For this review, take the finished solid that the model builds, in its own axes (mm). A direction names the side the tool comes from. Round coordinates to 2 decimals unless told otherwise and drop trailing zeros. Loops run counter-clockwise (first coordinate to the right, second up) from the corner with the lowest first, then second, coordinate; pieces in that order, holes last. Notation, with made-up numbers: (26, -26) -> (54, -26) arc R18 ccw to (54, -9) -> close; hole circle Ø3 at (58.5, -37). An arc over 180 degrees is marked (long way). One line per question, with ' | ' between items. Start each with the question number.
1. Consider section D-D (z = 1.5). Write out the cut boundary in (x, y), and give its area (3 significant figures).
2. Consider section C-C (y = 0). Write out the cut boundary in (x, z).
3. Consider section A-A (z = 5). Write out the cut boundary in (x, y).
4. Wall thickness on line 1 along Z through (x, y) = (6, -3); line 2 along Z through (x, y) = (13.5, -8); line 3 along Y through (x, z) = (0, 2.25): over which ranges is each line inside the solid? List them lowest first.
5. Draft analysis for pull direction X (two halves, no side actions). For faces 4 (the face through (14, -6, 2)), 5 (the face through (0, 0, 0)), state which applies: pulls with the +X half, pulls with the -X half, needs draft (parallel to the pull), parting line crosses it, or undercut.
6. For pin 1 Ø15 at (x, y) = (5.5, 4.5) entering from +Z; pin 2 Ø1.5 at (x, z) = (-9.5, 2) entering from -Y; pin 3 Ø2 at (x, z) = (9.5, 1.5) entering from +Y, all flat-tipped, find the tip position at first contact; note any pin that passes through.
7. For faces 1 (the face through (-12.1, -11.3, 4.5)), 2 (the face through (0, 0, 3)), 3 (the face through (12, -11.11, 7.51)), list the 3-axis set-ups (+Z, -Z, +X, -X, +Y, -Y) from which the entire face can be reached by the end or side of a thin tool; tool diameter is ignored.
8. Consider section B-B (x = 0). Write out the cut boundary in (y, z), and give its area (3 significant figures).
```python
from build123d import *

# Parameters (mm, degrees)
SKETCH1_R                                   = 17
SKETCH1_R_2                                 = 15
BOSS_EXTRUDE1_DEPTH                         = 2
SKETCH1_2_R                                 = 15
BOSS_EXTRUDE2_DEPTH                         = 3
BOSS_EXTRUDE3_DEPTH                         = 6
CUT_EXTRUDE1_START                          = -6
CUT_EXTRUDE1_DEPTH                          = 2.5
CHAMFER1_SIZE                               = 1
CHAMFER1_SIZE2                              = 0.2
CIRPATTERN1_COUNT                           = 2
CIRPATTERN1_ANGLE                           = 133
CHAMFER1_OF_CIRPATTERN1_SIZE2               = 0.2
CHAMFER1_OF_CIRPATTERN1_SIZE                = 1
CIRPATTERN1_THE_OTHER_WAY_COUNT             = 2
CIRPATTERN1_THE_OTHER_WAY_ANGLE             = 133
CHAMFER1_OF_CIRPATTERN1_THE_OTHER_WAY_SIZE2 = 0.2
CHAMFER1_OF_CIRPATTERN1_THE_OTHER_WAY_SIZE  = 1


with BuildPart() as part:
    # Sketch1 → Boss-Extrude1 (new body)
    with BuildSketch(Plane.XY):
        Circle(SKETCH1_R)
        Circle(SKETCH1_R_2, mode=Mode.SUBTRACT)
    extrude(amount=BOSS_EXTRUDE1_DEPTH)

    # Sketch1<2> → Boss-Extrude2 (add)
    with BuildSketch(Plane.XY):
        Circle(SKETCH1_2_R)
    extrude(amount=BOSS_EXTRUDE2_DEPTH)

    # Sketch2 → Boss-Extrude3 (add)
    with BuildSketch(Plane.XY.offset(2)):
        with BuildLine():
            ThreePointArc((4.184615385, 16.476923077), (0, 17), (-4.184615385, 16.476923077))
            Line((-4.184615385, 16.476923077), (-4, 15.75))
            ThreePointArc((-4, 15.75), (0, 16.25), (4, 15.75))
            Line((4, 15.75), (4.184615385, 16.476923077))
        make_face()
    boss_extrude3 = extrude(amount=BOSS_EXTRUDE3_DEPTH)

    # Sketch3 → Cut-Extrude1 (cut)
    with BuildSketch(Plane.XY.offset(8).offset(CUT_EXTRUDE1_START)):
        with BuildLine():
            ThreePointArc((1.25, 16.953981833), (0, 17), (-1.25, 16.953981833))
            Line((-1.25, 16.953981833), (-1.194852941, 16.206012046))
            ThreePointArc((-1.194852941, 16.206012046), (0, 16.25), (1.194852941, 16.206012046))
            Line((1.194852941, 16.206012046), (1.25, 16.953981833))
        make_face()
    cut_extrude1 = extrude(amount=CUT_EXTRUDE1_DEPTH, mode=Mode.SUBTRACT)

    # Chamfer1
    chamfer1_edges = [part.edges().sort_by_distance(p)[0] for p in [
        (0, 16.25, 8),
    ]]
    chamfer1_side = [part.faces().sort_by_distance(p)[0] for p in [
        (0, 16.25, 5),
    ]]
    chamfer(chamfer1_edges, length=CHAMFER1_SIZE, length2=CHAMFER1_SIZE2, reference=chamfer1_side[0])

    # CirPattern1: Boss-Extrude3, Cut-Extrude1 ×2 about axis
    cirpattern1_axis = Axis((0, 0, 0), (0, 0, -1))
    for i in range(1, CIRPATTERN1_COUNT):
        add(boss_extrude3.rotate(cirpattern1_axis, i * CIRPATTERN1_ANGLE / (CIRPATTERN1_COUNT - 1)))
        add(cut_extrude1.rotate(cirpattern1_axis, i * CIRPATTERN1_ANGLE / (CIRPATTERN1_COUNT - 1)), mode=Mode.SUBTRACT)

    # Chamfer1 of CirPattern1
    chamfer1_of_cirpattern1_edges = [part.edges().sort_by_distance(p)[0] for p in [
        (11.884497651, -11.082473351, 8),
    ]]
    chamfer(chamfer1_of_cirpattern1_edges, length=CHAMFER1_OF_CIRPATTERN1_SIZE, length2=CHAMFER1_OF_CIRPATTERN1_SIZE2)

    # CirPattern1 the other way: Boss-Extrude3, Cut-Extrude1 ×2 about axis
    cirpattern1_the_other_way_axis = Axis((0, 0, 0), (0, 0, 1))
    for i in range(1, CIRPATTERN1_THE_OTHER_WAY_COUNT):
        add(boss_extrude3.rotate(cirpattern1_the_other_way_axis, i * CIRPATTERN1_THE_OTHER_WAY_ANGLE / (CIRPATTERN1_THE_OTHER_WAY_COUNT - 1)))
        add(cut_extrude1.rotate(cirpattern1_the_other_way_axis, i * CIRPATTERN1_THE_OTHER_WAY_ANGLE / (CIRPATTERN1_THE_OTHER_WAY_COUNT - 1)), mode=Mode.SUBTRACT)

    # Chamfer1 of CirPattern1 the other way
    chamfer1_of_cirpattern1_the_other_way_edges = [part.edges().sort_by_distance(p)[0] for p in [
        (-11.884497651, -11.082473351, 8),
    ]]
    chamfer(chamfer1_of_cirpattern1_the_other_way_edges, length=CHAMFER1_OF_CIRPATTERN1_THE_OTHER_WAY_SIZE, length2=CHAMFER1_OF_CIRPATTERN1_THE_OTHER_WAY_SIZE2)


solid = part.part
```
Answer block:
1) outline: circle Ø34 at (0, 0) | area: 908 mm2
2) outline: (-17, 0) -> (17, 0) -> (17, 2) -> (15, 2) -> (15, 3) -> (-15, 3) -> (-15, 2) -> (-17, 2) -> close
3) outline: (-14.9, -8.18) arc R17 ccw to (-9.2, -14.3) -> (-8.79, -13.67) arc R16.25 cw to (-14.25, -7.82) -> close; (-4.18, 16.48) -> (-4, 15.75) arc R16.25 cw to (4, 15.75) -> (4.18, 16.48) arc R17 ccw to start; (8.79, -13.67) -> (9.2, -14.3) arc R17 ccw to (14.9, -8.18) -> (14.25, -7.82) arc R16.25 cw to start
4) line 1: z = 0 to 3 | line 2: z = 0 to 2 | line 3: y = -15 to 15
5) face 4: undercut | face 5: needs draft
6) pin 1: stops at z = 3 | pin 2: stops at y = -14.58 | pin 3: stops at y = 14.72
7) face 1: none | face 2: +Z | face 3: +Z, +Y
8) outline: (-17, 0) -> (17, 0) -> (17, 2) -> (15, 2) -> (15, 3) -> (-15, 3) -> (-15, 2) -> (-17, 2) -> close; (16.25, 4.5) -> (17, 4.5) -> (17, 8) -> (16.45, 8) -> (16.25, 7) -> close | area: 101 mm2
